```python
from build123d import *

# Parameters (mm, degrees)
SKETCH1_W           = 124.968
SKETCH1_H           = 99.568
BOSS_EXTRUDE1_DEPTH = 6.35
SKETCH2_R           = 44.45
BOSS_EXTRUDE2_DEPTH = 6.35
SKETCH3_W           = 44.45
SKETCH3_H           = 4.7625
BOSS_EXTRUDE3_DEPTH = 101.6
SKETCH4_R           = 4.7625
CUT_EXTRUDE1_DEPTH  = 80.9465
FILLET1_R           = 2.54


with BuildPart() as part:
    # Sketch1 → Boss-Extrude1 (new body)
    with BuildSketch(Plane(origin=(0, 0, 0), x_dir=(0, 0, -1), z_dir=(1, 0, 0))):
        with Locations((62.484, 49.784)):
            Rectangle(SKETCH1_W, SKETCH1_H)
    extrude(amount=BOSS_EXTRUDE1_DEPTH)

    # Sketch2 → Boss-Extrude2 (add)
    with BuildSketch(Plane(origin=(6.35, 0, 0), x_dir=(0, 0, -1), z_dir=(1, 0, 0))):
        with Locations((62.484, 49.784)):
            Circle(SKETCH2_R)
    extrude(amount=BOSS_EXTRUDE2_DEPTH)

    # Sketch3 → Boss-Extrude3 (add)
    with BuildSketch(Plane(origin=(12.7, 0, 0), x_dir=(0, 0, -1), z_dir=(1, 0, 0))):
        with Locations((62.484, 77.56525)):
            Rectangle(SKETCH3_W, SKETCH3_H)
        with Locations((62.484, 22.00275)):
            Rectangle(SKETCH3_W, SKETCH3_H)
    extrude(amount=BOSS_EXTRUDE3_DEPTH)

    # Sketch4 → Cut-Extrude1 (cut, through all)
    with BuildSketch(Plane.XZ.offset(-19.6215)):
        with Locations((101.6, -62.484)):
            Circle(SKETCH4_R)
    extrude(amount=-CUT_EXTRUDE1_DEPTH, mode=Mode.SUBTRACT)

    # Fillet1
    fillet1_edges = [part.edges().sort_by_distance(p)[0] for p in [
        (6.35, 49.784, -18.034),
        (12.7, 49.784, -18.034),
        (12.7, 77.56525, -40.259),
        (114.3, 77.56525, -84.709),
        (114.3, 77.56525, -40.259),
        (12.7, 22.00275, -84.709),
        (12.7, 22.00275, -40.259),
        (114.3, 22.00275, -84.709),
        (114.3, 22.00275, -40.259),
        (0, 49.784, 0),
        (3.175, 99.568, 0),
        (3.175, 99.568, -124.968),
        (3.175, 0, -124.968),
        (3.175, 0, 0),
    ]]
    fillet(fillet1_edges, radius=FILLET1_R)


solid = part.part
```
Design review of the part built by this model. Coordinates are the model's own, in mm. A direction names the side the tool comes from. Give positions to 0.01 mm unless a question says otherwise; leave off trailing zeros. Loops run counter-clockwise (first coordinate to the right, second up) from the corner with the lowest first, then second, coordinate; pieces in that order, holes last. Notation, with made-up numbers: (-4, 18.25) -> (44, 18.25) arc R12 cw to (44, 29.25) -> close; hole circle Ø2 at (4.5, -36). An arc over 180 degrees is marked (long way). One line per item, written item: value.
Q1. Machinability: for faces 1 (the flat face through (63, 78, -40.259)), 2 (the cylindrical face through (9.5, 79.8, -29.7)), 3 (the flat face through (63, 19.621, -62)), 4 (the flat face through (63, 75.184, -61)), 5 (the flat face through (114.3, 22, -62)), which of the approach directions +Z, -Z, +X, -X, +Y, -Y give a long, thin tool a straight path to every point of the face, cutting with its end or side? Answer none if there is none.
Numbers:
face 1: +Z, +X, +Y, -Y
face 2: +X
face 3: +Z, -Z, +X, -Y
face 4: +Z, -Z, +X
face 5: +Z, -Z, +X, +Y, -Y
Q2. We need section A-A on x = 101.6. Give the boundary of the cut face in (y, z), and give its area (3 significant figures).
Numbers:
outline: (19.62, -84.71) -> (24.38, -84.71) -> (24.38, -67.25) -> (19.62, -67.25) -> close; (19.62, -57.72) -> (24.38, -57.72) -> (24.38, -40.26) -> (19.62, -40.26) -> close; (75.18, -84.71) -> (79.95, -84.71) -> (79.95, -67.25) -> (75.18, -67.25) -> close; (75.18, -57.72) -> (79.95, -57.72) -> (79.95, -40.26) -> (75.18, -40.26) -> close
area: 333 mm^2
Q3. We need section B-B on x = 65. Give the boundary of the cut face in (y, z).
Numbers:
outline: (19.62, -84.71) -> (24.38, -84.71) -> (24.38, -40.26) -> (19.62, -40.26) -> close; (75.18, -84.71) -> (79.95, -84.71) -> (79.95, -40.26) -> (75.18, -40.26) -> close
Q4. Draft analysis for pull direction Y (two halves, no side actions). For faces 6 (the flat face through (63, 24.384, -62)), 7 (the cylindrical face through (98.09, 21.969, -59.265)), 8 (the flat face through (63, 79.946, -61)), state which applies: pulls with the +Y half, pulls with the -Y half, needs draft (parallel to the pull), parting line crosses it, or undercut.
Numbers:
face 6: undercut
face 7: needs draft
face 8: pulls with the +Y half
Q5. For pin 1 Ø5 at (x, y) = (48.5, 77.5) entering from +Z; pin 2 Ø23.5 at (x, z) = (45, -55) entering from +Y; pin 3 Ø1.4 at (x, y) = (61, 22.5) entering from -Z, all flat-tipped, find the tip position at first contact; note any pin that passes through.
Numbers:
pin 1: stops at z = -40.26
pin 2: stops at y = 79.95
pin 3: stops at z = -84.71
Q6. For L1, parallel to Y at x = 30.5, z = -72; L2, parallel to Z at x = 101.6, y = 77.55; L3, parallel to Z at x = 101, y = 22, list the stretches that pass through material, from the lowest coordinate up.
Numbers:
L1: y = 19.62 to 24.38, 75.18 to 79.95
L2: z = -84.71 to -67.25, -57.72 to -40.26
L3: z = -84.71 to -67.21, -57.76 to -40.26
